```python
from build123d import *

# Parameters (mm, degrees)
BOSS_EXTRUDE1_DEPTH = 8
SKETCH2_R           = 2
CUT_EXTRUDE1_DEPTH  = 13


with BuildPart() as part:
    # Sketch1 → Boss-Extrude1 (new body)
    with BuildSketch(Plane.XY):
        with BuildLine():
            Line((-7.885993485, 10.084690554), (-7.885993485, -1.915309446))
            Line((-7.885993485, -1.915309446), (19.114006515, -1.915309446))
            Line((19.114006515, -1.915309446), (19.114006515, 10.084690554))
            Line((19.114006515, 10.084690554), (12.614006515, 10.084690554))
            ThreePointArc((12.614006515, 10.084690554), (5.614006515, 3.084690554), (-1.385993485, 10.084690554))
            Line((-1.385993485, 10.084690554), (-7.885993485, 10.084690554))
        make_face()
    extrude(amount=BOSS_EXTRUDE1_DEPTH)

    # Sketch2 → Cut-Extrude1 (cut, through all)
    with BuildSketch(Plane(origin=(0, 10.084690554, 0), x_dir=(1, 0, 0), z_dir=(0, 1, 0))):
        with Locations((-3.885993485, -4)):
            Circle(SKETCH2_R)
        with Locations((15.114006515, -4)):
            Circle(SKETCH2_R)
    extrude(amount=-CUT_EXTRUDE1_DEPTH, mode=Mode.SUBTRACT)


solid = part.part
```
Input: part model. Units: mm. Frame: model coordinates. Coordinates: 2 decimals unless noted, no trailing zeros. Write each loop counter-clockwise with the first axis right and the second up, starting at its lowest first coordinate (ties: lowest second). Pieces come first, ordered by that corner, then holes.
1) Pin query (flat end, axial travel): pin 1 Ø3 at (x, y) = (16, 6) entering from -Z. Return the tip coordinate at first contact, or that it passes through.
2) Section B-B on y = 5.25. Output: boundary loops of the cut face in (x, z), and give its area (3 significant figures).
3) Section D-D on z = 1.25. Output: boundary loops of the cut face in (x, y), and give its area (3 significant figures).
4) Material intervals for line 1 along X through (y, z) = (-1.5, 3.75); line 2 along X through (y, z) = (9, 4.5); line 3 along X through (y, z) = (5.5, 1.75), sorted ascending.
5) Section C-C on y = 0.25. Output: boundary loops of the cut face in (x, z), and give its area (3 significant figures).
6) Section A-A on z = 4. Output: boundary loops of the cut face in (x, y).
7) Mould query, pull axis X, two halves, no side actions, for faces 1 (the flat face through (19.114, 4, 4)), 2 (the cylindrical face through (13.116, 4.169, 3.912)), 3 (the flat face through (5.4, 2.8, 8)). Classes: pulls with the +X half, pulls with the -X half, needs draft (parallel to the pull), parting line crosses it, or undercut.
Check result:
1. pin 1: stops at z = 0
2. outline: (-7.89, 0) - (0.55, 0) - (0.55, 8) - (-7.89, 8) - close; (10.68, 0) - (19.11, 0) - (19.11, 8) - (10.68, 8) - close; hole circle Ø4 at (-3.89, 4); hole circle Ø4 at (15.11, 4)
2. area: 110 mm2
3. outline: (-7.89, -1.92) - (19.11, -1.92) - (19.11, 10.08) - (12.61, 10.08) arc R7 cw to (-1.39, 10.08) - (-7.89, 10.08) - close
3. area: 247 mm2
4. line 1: x = -7.89 to -5.87, -1.9 to 13.13, 17.1 to 19.11
4. line 2: x = -7.89 to -5.82, -1.95 to -1.3, 12.53 to 13.18, 17.05 to 19.11
4. line 3: x = -7.89 to 0.32, 10.9 to 19.11
5. outline: (-7.89, 0) - (19.11, 0) - (19.11, 8) - (-7.89, 8) - close; hole circle Ø4 at (-3.89, 4); hole circle Ø4 at (15.11, 4)
5. area: 191 mm2
6. outline: (-7.89, -1.92) - (-5.89, -1.92) - (-5.89, 10.08) - (-7.89, 10.08) - close; (-1.89, -1.92) - (13.11, -1.92) - (13.11, 10.08) - (12.61, 10.08) arc R7 cw to (-1.39, 10.08) - (-1.89, 10.08) - close; (17.11, -1.92) - (19.11, -1.92) - (19.11, 10.08) - (17.11, 10.08) - close
7. face 1: pulls with the +X half
7. face 2: undercut
7. face 3: needs draft
